Autodesk Inventor part; units mm, degrees
ref_plane "YZ Plane" through (0, 0, 0) normal (1, 0, 0) x (0, 1, 0)
ref_plane "XZ Plane" through (0, 0, 0) normal (0, 1, 0) x (-1, 0, 0)
ref_plane "XY Plane" through (0, 0, 0) normal (0, 0, 1) x (1, 0, 0)
sketch "Sketch1" plane through (0, 0, 0) normal (0, 1, 0) x (-1, 0, 0)
  line L0 (12.7, 6.985) -> (-12.7, 6.985)
  line L1 (-12.7, 6.985) -> (-12.7, -6.985)
  line L2 (-12.7, -6.985) -> (12.7, -6.985)
  line L3 (12.7, -6.985) -> (12.7, 6.985)
  point P0 (0, 0)
  dimension "depth" = 25.4
  dimension "width" = 13.97
  dimension "d5" = 6.985
  dimension "d6" = 12.7
extrude "body" add sketch "Sketch1" along normal blind 19.05
sketch "Sketch3" plane through (12.7, 0, 6.985) normal (1, 0, 0) x (0, 0, -1)
  point P0 (6.985, 0)
sketch "Sketch5" plane through (0, 19.05, 0) normal (0, 1, 0) x (1, 0, 0)
  line L0 (-12.7, -6.985) -> (12.7, -6.985)
  point P0 (0, 0)
  point P1 (0, -4.699)
  dimension "d25" = 0
  dimension "d34" = 6.985
  dimension "hole_radius" = 2.286
hole "main odor hole" at (0, 19.05, 4.699) direction (0, -1, 0) diameter 4.2291 depth 14.732 tip angle 118
sketch "Sketch6" plane through (-12.7, 0, 6.985) normal (0, 0, 1) x (1, 0, 0)
  line L0 (0, 0) -> (25.4, 0)
  point P0 (12.7, 0)
  point P1 (15.2082, 15.494)
  point P2 (10.1917, 15.494)
  dimension "d126" = 15.494
  dimension "d127" = 5.0165
  dimension "d128" = 2.5082
hole "lickports" at (2.5083, 15.494, 6.985) at (-2.5082, 15.494, 6.985) direction (0, 0, -1) diameter 0.7112 end through all
sketch "Sketch7" plane through (12.7, 0, -6.985) normal (0, 0, -1) x (-1, 0, 0)
  line L0 (14.8146, 4.318) -> (10.5855, 4.318)
  point P0 (12.7, 0)
  point P1 (12.7, 4.318)
hole "fitting threads" at (0, 4.318, -6.985) direction (0, 0, 1) diameter 5.3594 depth 6.35
sketch "Sketch8" plane through (0, 4.318, -0.635) normal (0, 0, -1) x (-1, 0, 0)
  line L0 (2.1146, 0) -> (-2.1145, 0)
  point P0 (0, -4.318)
  point P1 (0, 0)
hole "input odor hole" at (0, 4.318, -0.635) direction (0, 0, 1) diameter 0.7937 depth 5.08
sketch "Sketch9" plane through (-12.7, 0, 6.985) normal (0, 0, 1) x (1, 0, 0)
  line L0 (0, 0) -> (25.4, 0)
  point P0 (12.7, 0)
  point P1 (12.7, 8.636)
  point P2 (12.7, 0)
  dimension "nose_hole" = 8.636
hole "nose_hole" at (0, 8.636, 6.985) direction (0, 0, -1) diameter 4.445 depth 4.1148 tip angle 110
sketch "Sketch10" plane through (0, 19.05, 0) normal (0, 1, 0) x (1, 0, 0)
  point P0 (0, 0)
  point P1 (7.9375, 2.54)
  point P2 (-7.9375, 2.54)
  dimension "d70" = 2.54
  dimension "d116" = 15.875
  dimension "d117" = 7.9375
hole "mount holes" at (7.9375, 19.05, -2.54) at (-7.9375, 19.05, -2.54) direction (0, -1, 0) diameter 2.6416 depth 10.16 tip angle 118
sketch "Sketch11" plane through (12.7, 0, -6.985) normal (0, 0, -1) x (-1, 0, 0)
  line L0 (0, 19.05) -> (25.4, 19.05)
  line L1 (0, 0) -> (25.4, 0)
  point P0 (12.7, 0)
  point P1 (12.7, 13.208)
  point P2 (12.7, 0)
  dimension "vacuum_height" = 5.842
hole "exhaust threading" at (0, 13.208, -6.985) direction (0, 0, 1) diameter 3.9624 depth 6.35
sketch "Sketch12" plane through (0, 13.208, -0.635) normal (0, 0, -1) x (-1, 0, 0)
  line L0 (-12.7, -13.208) -> (12.7, -13.208)
  line L1 (-12.7, 5.842) -> (12.7, 5.842)
  point P0 (0, -13.208)
  point P1 (0, 0)
  point P2 (0, -13.208)
  dimension "d87" = 5.842
hole "exhaust hole" at (0, 13.208, -0.635) direction (0, 0, 1) diameter 1.5875 depth 5.08
sketch "Sketch16" plane through (12.7, 0, -6.985) normal (0, 0, -1) x (-1, 0, 0)
  circle A0 centre (12.7, 8.636) radius 2.9083
  line L0 (15.6083, 8.636) -> (12.7, 8.636)
  point P0 (12.7, 0)
hole "sniff_monitoring_hole" at (0, 8.636, -6.985) direction (0, 0, 1) diameter 0.7112 end through all
fillet "nose hole fillet" [suppressed]
sketch "Sketch25" plane through (12.7, 0, 6.985) normal (1, 0, 0) x (0, 0, -1)
  line L0 (7.62, 1.6383) -> (7.62, 6.9977)
  point P0 (6.985, 0)
  point P1 (7.62, 4.318)
  point P2 (6.5343, 4.318)
  point P3 (4.363, 4.318)
  dimension "d147" = 3.257
  dimension "d148" = 1.0857
hole "vac fitting" at (12.7, 4.318, 0.4507) direction (-1, 0, 0) diameter 3.9624 depth 6.35
hole "vac hole" at (6.35, 4.318, 0.4507) direction (-1, 0, 0) diameter 0.7937 depth 6.35 tip angle 118
chamfer "front panel chamfer" distance 6.858 angle 30 2 edges at (12.7, 9.525, 6.985) (-12.7, 9.525, 6.985) measured on face at (9.2021, 9.318, 6.985)
fillet "Fillet4" radius 0.381 1 edges at (0, 10.8585, 6.985)
equation "\"d27\" = 1.85 * hole_radius"
equation "\"d29\" = 2 * hole_radius"
equation "\"d66\" = 1.8 * hole_radius"
equation "\"d150\" = vac_thread_depth"
equation "\"d154\" = vac_fit_depth"
properties part number "odorport_final_wvac"
For this review, take the finished solid that the model builds, in its own axes (mm). A direction names the side the tool comes from. Give positions to 0.01 mm unless a question says otherwise; leave off trailing zeros. Order: outer loops, then holes, each group sorted by start corner. A loop starts at its lowest first (then second) coordinate and runs counter-clockwise, first axis right, second up. Notation, with made-up numbers: (-12, 2.5) - (21, 2.5) arc R13 ccw to (21, 20.5) - close; hole circle Ø11 at (88, 55). An arc over 180 degrees is marked (long way). Answer as a JSON object with one key per item and string values. Group by question number.
Item 1: Take a section at C-C on y = 2. Give the boundary of the cut face in (x, z) (1 decimal), and give its area (3 significant figures).
Item 2: Wall thickness on line 1 along Y through (x, z) = (0, -4); line 2 along X through (y, z) = (15.5, -5.25); line 3 along Z through (x, y) = (0, 15) (3 decimals): over which ranges is each line inside the solid? List them lowest first.
Item 3: Machinability: for faces 1 (the cylindrical face through (9.481, 2.354, 0.709)), 2 (the flat face through (0, 19.05, 0)), 3 (the cylindrical face through (-0.035, 12.415, 1.076)), 4 (the flat face through (9.319, 9.658, 4.978)), 5 (the cylindrical face through (0.81, 14.117, 6.652)), which of the approach directions +Z, -Z, +X, -X, +Y, -Y give a long, thin tool a straight path to every point of the face, cutting with its end or side? Answer none if there is none.
Item 4: Clearance check with flat-ended pins moving along their axes: pin 1 Ø1 at (y, z) = (3, 4.5) entering from +X; pin 2 Ø1.2 at (y, z) = (5, 1.5) entering from +X; pin 3 Ø2.5 at (x, y) = (0, 4.5) entering from -Z (3 decimals). State where each tip first meets the part, or that it passes through.
Item 5: Take a section at A-A on z = -5.75. Give the boundary of the cut face in (x, y).
Item 6: Take a section at D-D on z = 6.25. Give the number of separate pieces and of enclosed holes in the cut face, and give its area (3 significant figures).
Item 7: Draft analysis for pull direction Y (two halves, no side actions). For faces 6 (the cylindrical face through (2.222, 8.672, 4.711)), 7 (the flat face through (-9.319, 9.392, 4.978)), 8 (the flat face through (0, 0, 0)), state which applies: pulls with the +Y half, pulls with the -Y half, needs draft (parallel to the pull), parting line crosses it, or undercut.
Reported:
{
 "1": {"outline": "(-12.7, -7) - (-1.3, -7) - (-1.3, -0.6) - (1.3, -0.6) - (1.3, -7) - (12.7, -7) - (12.7, 3) - (5.8, 7) - (-5.8, 7) - (-12.7, 3) - close", "area": "311 mm^2"},
 "2": {"line 1": "0 to 1.64, 7 to 8.28, 8.99 to 11.23, 15.19 to 19.05", "line 2": "-12.7 to -2.86, -2.15 to 2.15, 2.86 to 12.7", "line 3": "-0.635 to 2.584, 6.814 to 6.985"},
 "3": {"face 1": "+X", "face 2": "+Z, -Z, +X, -X, +Y", "face 3": "-Z", "face 4": "+Z, +X, +Y, -Y", "face 5": "+Y"},
 "4": {"pin 1": "x = 11.01", "pin 2": "x = 6.35", "pin 3": "z = -0.635"},
 "5": {"outline": "(-12.7, 0) - (12.7, 0) - (12.7, 19.05) - (-12.7, 19.05) - close; hole circle Ø0.71 at (-2.51, 15.49); hole circle Ø5.36 at (0, 4.32); hole circle Ø3.96 at (0, 13.21); hole circle Ø0.71 at (0, 8.64); hole circle Ø0.71 at (2.51, 15.49)"},
 "6": {"separate pieces": "1", "enclosed holes": "2", "area": "224 mm^2"},
 "7": {"face 6": "undercut", "face 7": "needs draft", "face 8": "pulls with the -Y half"}
}
